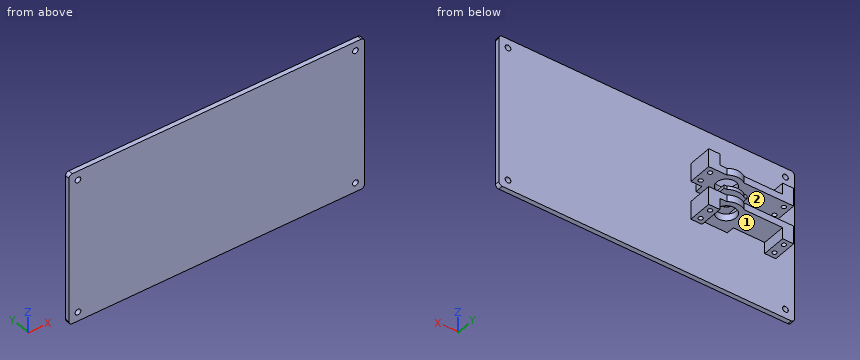
```python
from build123d import *

# Parameters (mm, degrees)
SKETCH_1_W                      = 260
SKETCH_1_H                      = 135
EXTRUDE_1_DEPTH                 = 4
HOLE_WIZARD_5_0_5_1_D           = 5
HOLE_WIZARD_5_0_5_1_CSINK_D     = 5.05
HOLE_WIZARD_5_0_5_1_CSINK_ANGLE = 90
FILLET_1_R                      = 3
EXTRUDE_2_DEPTH                 = 15
SKETCH_5_W                      = 5
SKETCH_5_H                      = 30.479983875
SKETCH_5_W_2                    = 10
CUT_EXTRUDE_2_DEPTH             = 251.053170719
SKETCH_7_W                      = 41.194630643
SKETCH_7_H                      = 3
CUT_EXTRUDE_3_DEPTH             = 20.987549798
SKETCH_8_W                      = 13.542667964
SKETCH_8_H                      = 3
CUT_EXTRUDE_5_DEPTH             = 28.013263597
SKETCH_9_W                      = 3.853145938
SKETCH_9_H                      = 3
CUT_EXTRUDE_6_DEPTH             = 7.025713799
SKETCH_11_W                     = 9.744219549
SKETCH_11_H                     = 20.987549798
EXTRUDE_3_DEPTH                 = 10
SKETCH_12_W                     = 9.744219549
SKETCH_12_H                     = 20.987549798
EXTRUDE_4_DEPTH                 = 10
SKETCH_13_R                     = 1.907696141
CUT_EXTRUDE_7_DEPTH             = 164.233327749
SKETCH_15_R                     = 8.546756312
CUT_EXTRUDE_8_DEPTH             = 10
EXTRUDE_5_DEPTH                 = 5
EXTRUDE_5_DEPTH_BACK            = 5
SKETCH_16_R                     = 4.379825861
FILLET_2_R                      = 3


with BuildPart() as part:
    # 草图1 → 凸台-拉伸1 (new body)
    with BuildSketch(Plane(origin=(0, 0, 0), x_dir=(1, 0, 0), z_dir=(0, 1, 0))):
        Rectangle(SKETCH_1_W, SKETCH_1_H)
    extrude(amount=EXTRUDE_1_DEPTH)

    # Ø5.0 (5) 直径孔1 (through all)
    with Locations(Plane(origin=(0, 4, 0), x_dir=(1, 0, 0), z_dir=(0, 1, 0))):
        with Locations((-122, 59.5), (-122, -59.5), (122, -59.5), (122, 59.5)):
            CounterSinkHole(HOLE_WIZARD_5_0_5_1_D / 2, HOLE_WIZARD_5_0_5_1_CSINK_D / 2, counter_sink_angle=HOLE_WIZARD_5_0_5_1_CSINK_ANGLE)

    # 圆角1
    fillet_1_edges = [part.edges().sort_by_distance(p)[0] for p in [
        (130, 2, 67.5),
        (-130, 2, 67.5),
        (-130, 2, -67.5),
        (130, 2, -67.5),
    ]]
    fillet(fillet_1_edges, radius=FILLET_1_R)

    # 草图4 → 凸台-拉伸2 (add, symmetric)
    with BuildSketch(Plane.XY):
        with BuildLine():
            Line((-70.947140493, 4), (-43.349875336, 4))
            Line((-43.349875336, 4), (-43.349875336, 11.025713799))
            Line((-43.349875336, 11.025713799), (-33.605655787, 11.025713799))
            Line((-33.605655787, 11.025713799), (-33.605655787, 32.013263597))
            Line((-33.605655787, 32.013263597), (-43.349875336, 32.013263597))
            Line((-43.349875336, 32.013263597), (-49.476243699, 32.013263597))
            ThreePointArc((-49.476243699, 32.013263597), (-57.148507914, 34.479983875), (-64.82077213, 32.013263597))
            Line((-64.82077213, 32.013263597), (-98.544405649, 32.013263597))
            Line((-98.544405649, 32.013263597), (-108.288625198, 32.013263597))
            Line((-108.288625198, 32.013263597), (-108.288625198, 11.025713799))
            Line((-108.288625198, 11.025713799), (-98.544405649, 11.025713799))
            Line((-98.544405649, 11.025713799), (-70.947140493, 11.025713799))
            Line((-70.947140493, 11.025713799), (-70.947140493, 4))
        make_face()
    extrude(amount=EXTRUDE_2_DEPTH, both=True)

    # 草图5 → 切除-拉伸2 (cut, through all)
    with BuildSketch(Plane.ZY.offset(108.288625198)):
        with Locations((-6.5, 19.239991938)):
            Rectangle(SKETCH_5_W, SKETCH_5_H)
        with Locations((4, 19.239991938)):
            Rectangle(SKETCH_5_W_2, SKETCH_5_H)
    extrude(amount=-CUT_EXTRUDE_2_DEPTH, mode=Mode.SUBTRACT)

    # 草图7 → 切除-拉伸3 (cut)
    with BuildSketch(Plane(origin=(0, 32.013263597, 0), x_dir=(1, 0, 0), z_dir=(0, 1, 0))):
        with Locations((-87.691309877, 2.5)):
            Rectangle(SKETCH_7_W, SKETCH_7_H)
    extrude(amount=-CUT_EXTRUDE_3_DEPTH, mode=Mode.SUBTRACT)

    # 草图8 → 切除-拉伸5 (cut)
    with BuildSketch(Plane(origin=(0, 32.013263597, 0), x_dir=(1, 0, 0), z_dir=(0, 1, 0))):
        with Locations((-40.376989769, 2.5)):
            Rectangle(SKETCH_8_W, SKETCH_8_H)
    extrude(amount=-CUT_EXTRUDE_5_DEPTH, mode=Mode.SUBTRACT)

    # 草图9 → 切除-拉伸6 (cut)
    with BuildSketch(Plane(origin=(0, 11.025713799, 0), x_dir=(1, 0, 0), z_dir=(0, 1, 0))):
        with Locations((-69.020567524, 2.5)):
            Rectangle(SKETCH_9_W, SKETCH_9_H)
    extrude(amount=-CUT_EXTRUDE_6_DEPTH, mode=Mode.SUBTRACT)

    # 草图11 → 凸台-拉伸3 (add)
    with BuildSketch(Plane.XY.offset(15)):
        with Locations((-38.477765562, 21.519488698)):
            Rectangle(SKETCH_11_W, SKETCH_11_H)
        with Locations((-103.416515424, 21.519488698)):
            Rectangle(SKETCH_11_W, SKETCH_11_H)
    extrude(amount=EXTRUDE_3_DEPTH)

    # 草图12 → 凸台-拉伸4 (add)
    with BuildSketch(Plane(origin=(0, 0, -15), x_dir=(-1, 0, 0), z_dir=(0, 0, -1))):
        with Locations((38.477765562, 21.519488698)):
            Rectangle(SKETCH_12_W, SKETCH_12_H)
        with Locations((103.416515424, 21.519488698)):
            Rectangle(SKETCH_12_W, SKETCH_12_H)
    extrude(amount=EXTRUDE_4_DEPTH)

    # 草图13 → 切除-拉伸7 (cut, through all)
    with BuildSketch(Plane.XY.offset(25)):
        with Locations(Location((-38.477765562, 27.075045448, 0), (0, 0, 90))):
            Circle(SKETCH_13_R)
        with Locations(Location((-38.477765562, 15.963931947, 0), (0, 0, 90))):
            Circle(SKETCH_13_R)
        with Locations((-103.416515423, 15.963931947)):
            Circle(SKETCH_13_R)
        with Locations((-103.416515423, 27.075045448)):
            Circle(SKETCH_13_R)
    extrude(amount=-CUT_EXTRUDE_7_DEPTH, mode=Mode.SUBTRACT)

    # 草图15 → 切除-拉伸8 (cut)
    with BuildSketch(Plane.XY.offset(15)):
        with Locations((-57.148507914, 21.315064512)):
            Circle(SKETCH_15_R)
    cut_extrude_8 = extrude(amount=-CUT_EXTRUDE_8_DEPTH, mode=Mode.SUBTRACT)

    # 镜向3: 切除-拉伸8 across plane
    add(cut_extrude_8.mirror(Plane.XY), mode=Mode.SUBTRACT)

    # 草图16 → 凸台-拉伸5 (add, two sides: drawn at the far end of the back side and taken through both)
    with BuildSketch(Plane.XY.offset(-1).offset(-EXTRUDE_5_DEPTH_BACK)):
        with Locations((-57.148507914, 21.315064512)):
            Circle(SKETCH_16_R)
    extrude(amount=EXTRUDE_5_DEPTH + EXTRUDE_5_DEPTH_BACK)

    # 圆角2
    fillet_2_edges = [part.edges().sort_by_distance(p)[0] for p in [
        (-57.121159153, 4, -4),
        (-57.121159153, 4, -1),
    ]]
    fillet(fillet_2_edges, radius=FILLET_2_R)


solid = part.part
```
Could you check a few things on this model? Use its own coordinates, in mm. Face numbers are marked on the shaded views. Coordinates: 2 decimals unless noted, no trailing zeros. Order: outer loops, then holes, each group sorted by start corner. A loop starts at its lowest first (then second) coordinate and runs counter-clockwise, first axis right, second up. Notation, with made-up numbers: M 69.5,-20.5 L 105.5,-20.5 A29 ccw 105.5,17.5 Z; hole C -9,7.5 d1. An arc over 180 degrees is marked long. Use a Markdown table: item, result. Add a question column.
Q1. I want a section at B-B on z = -59.5. List the corners of the cut face in (x, y) for me (3 decimals).
Q2. I'm going to push flat-ended pins straight in: pin 1 (8 mm diameter, centred on x = -70.5, y = 28.5, fed in from -Z); pin 2 (5 mm diameter, centred on x = -95, z = 14.5, fed in from +Y); pin 3 (2.5 mm diameter, centred on x = -56, y = 21.5, fed in from +Z). Where does each tip first touch, or does it pass through?
Q3. I want a section at A-A on x = -122. List the corners of the cut face in (y, z) for me (3 decimals), then the cut area to 3 significant figures.
Q4. If I drill on L1, parallel to Z at x = 122, y = 2.55; L2, parallel to X at y = 3, z = -59.5; L3, parallel to X at y = 2, z = -59, over which ranges is the centre line in solid material (lowest first)?
Q5. We'd pull the mould along X, two halves only. Please class the marked faces 1 and 2: pulls with the +X half, pulls with the -X half, needs draft (parallel to the pull), parting line crosses it, or undercut.
Q6. I want a section at C-C on z = -21. List the corners of the cut face in (x, y) for me.
Checked values:
| question | item | result |
|---|---|---|
| 1 | outline | M -130,0 L -124.5,0 L -124.5,3.975 L -124.525,4 L -130,4 Z; M -119.5,0 L 119.5,0 L 119.5,3.975 L 119.475,4 L -119.475,4 L -119.5,3.975 Z; M 124.5,0 L 130,0 L 130,4 L 124.525,4 L 124.5,3.975 Z |
| 2 | pin 1 | z = -15 |
| 2 | pin 2 | y = 32.01 |
| 2 | pin 3 | z = 4 |
| 3 | outline | M 0,-67.5 L 4,-67.5 L 4,-62.025 L 3.975,-62 L 0,-62 Z; M 0,-57 L 3.975,-57 L 4,-56.975 L 4,56.975 L 3.975,57 L 0,57 Z; M 0,62 L 3.975,62 L 4,62.025 L 4,67.5 L 0,67.5 Z |
| 3 | area | 500 mm² |
| 4 | L1 | -67.5 to -62, -57 to 57, 62 to 67.5 |
| 4 | L2 | -130 to -124.5, -119.5 to 119.5, 124.5 to 130 |
| 4 | L3 | -130 to -124.45, -119.55 to 119.55, 124.45 to 130 |
| 5 | face 1 | undercut |
| 5 | face 2 | needs draft |
| 6 | outline | M -130,0 L 130,0 L 130,4 L -130,4 Z; M -108.29,11.03 L -98.54,11.03 L -98.54,32.01 L -108.29,32.01 Z; M -43.35,11.03 L -33.61,11.03 L -33.61,32.01 L -43.35,32.01 Z; hole C -103.42,15.96 d3.82; hole C -103.42,27.08 d3.82; hole C -38.48,15.96 d3.82; hole C -38.48,27.08 d3.82 |
